```python
from build123d import *

# Parameters (mm, degrees)
F1_DEPTH = 1.8
F3_DEPTH = 1.5
F4_R     = 1.5
F5_DEPTH = 3.3
F6_R     = 3


with BuildPart() as f1:
    # F0 (on Top) → F1 (new body)
    with BuildSketch(Plane.XY):
        Polygon((18.5, 14), (-14, 14), (-14, -14), (18.5, -14), (18.5, -7), (-7, -7), (-7, 7), (18.5, 7), align=None)
    extrude(amount=F1_DEPTH)

    # F2 (on face) → F3 (join)
    with BuildSketch(Plane.XY.offset(1.8)):
        Polygon((-9, -9), (-9, 9), (13.6, 9), (13.6, 7), (18.5, 7), (18.5, 14), (-14, 14), (-14, -14), (18.5, -14), (18.5, -7), (13.6, -7), (13.6, -9), align=None)
    extrude(amount=F3_DEPTH)

    # F4 (on face) → F5 (cut, through all)
    with BuildSketch(Plane.XY.offset(3.3)):
        with Locations((-11, 11)):
            Circle(F4_R)
        with Locations((15.5, 11)):
            Circle(F4_R)
        with Locations((15.5, -11)):
            Circle(F4_R)
        with Locations((-11, -11)):
            Circle(F4_R)
    extrude(amount=-F5_DEPTH, mode=Mode.SUBTRACT)

    # F6
    f6_edges = [f1.edges().sort_by_distance(p)[0] for p in [
        (-14, -14, 1.65),
        (18.5, -14, 1.65),
        (18.5, 14, 1.65),
        (-14, 14, 1.65),
    ]]
    fillet(f6_edges, radius=F6_R)


solid = f1.part
```
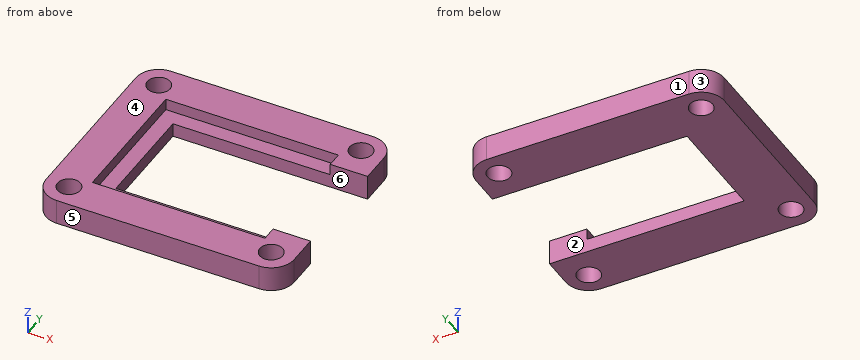
Verification items for the finished model (mm, model axes). Face numbers are marked on the shaded views. A direction names the side the tool comes from. Coordinates: 2 decimals unless noted, no trailing zeros. Write each loop counter-clockwise with the first axis right and the second up, starting at its lowest first coordinate (ties: lowest second). Pieces come first, ordered by that corner, then holes. Notation, with made-up numbers: (-11.75, 50) - (14.25, 50) arc R5 cw to (14.25, 56) - close; hole circle Ø4 at (-36, 78.5). An arc over 180 degrees is marked (long way). One line per question, with ' | ' between items. Start each with the question number.
1. Gauge pin test, flat ends, axial feed: P1, Ø0.9, axis at y = -3.5, z = 1, coming from the +X side; P2, Ø5, axis at x = -0.5, y = 9, coming from the -Z side; P3, Ø2.5, axis at x = -11, y = -11, coming from the +Z side; P4, Ø1.6, axis at y = 1.5, z = 3, coming from the +X side. Record the tip position at first contact, or that the pin passes through.
2. Section check A-A (x = 9). Enter the section's corners in (y, z), plus the area to 3 significant figures.
3. Access from +Z, -Z, +X, -X, +Y, -Y to the whole of each face (thin tool, end or side, straight path). Record for the marked faces 1 and 2.
4. Draft check along Y on the marked faces 3, 4, 5 and 6. Enter one of: released by +Y, released by -Y, zero draft, split by the parting line, or undercut.
5. Section check B-B (y = -11.75). Enter the section's corners in (x, z).
6. Section check D-D (y = 8). Enter the section's corners in (x, z), plus the area to 4 significant figures.
7. Section check C-C (z = 0.95). Enter the section's corners in (x, y).
8. Material ranges on line 1 along Y through (x, z) = (15.5, 2.15); line 2 along Y through (x, z) = (-11, 2.6); line 3 along Y through (x, z) = (1, 0.35), recorded low to high.
Computed values:
1) P1: x = -7 | P2: z = 0 | P3: through | P4: x = -9
2) outline: (-14, 0) - (-7, 0) - (-7, 1.8) - (-9, 1.8) - (-9, 3.3) - (-14, 3.3) - close; (7, 0) - (14, 0) - (14, 3.3) - (9, 3.3) - (9, 1.8) - (7, 1.8) - close | area: 40.2 mm²
3) face 1: +Z, -Z, +X, -X, +Y | face 2: +Z, -Z, +X
4) face 3: released by +Y | face 4: zero draft | face 5: released by -Y | face 6: undercut
5) outline: (-13.9, 0) - (-12.3, 0) - (-12.3, 3.3) - (-13.9, 3.3) - close; (-9.7, 0) - (14.2, 0) - (14.2, 3.3) - (-9.7, 3.3) - close; (16.8, 0) - (18.4, 0) - (18.4, 3.3) - (16.8, 3.3) - close
6) outline: (-14, 0) - (18.5, 0) - (18.5, 3.3) - (13.6, 3.3) - (13.6, 1.8) - (-9, 1.8) - (-9, 3.3) - (-14, 3.3) - close | area: 73.35 mm²
7) outline: (-14, -11) arc R3 ccw to (-11, -14) - (15.5, -14) arc R3 ccw to (18.5, -11) - (18.5, -7) - (-7, -7) - (-7, 7) - (18.5, 7) - (18.5, 11) arc R3 ccw to (15.5, 14) - (-11, 14) arc R3 ccw to (-14, 11) - close; hole circle Ø3 at (-11, -11); hole circle Ø3 at (-11, 11); hole circle Ø3 at (15.5, -11); hole circle Ø3 at (15.5, 11)
8) line 1: -14 to -12.5, -9.5 to -7, 7 to 9.5, 12.5 to 14 | line 2: -14 to -12.5, -9.5 to 9.5, 12.5 to 14 | line 3: -14 to -7, 7 to 14
